from build123d import *

# Parameters (mm, degrees)
SKETCH1_W                = 20
SKETCH1_H                = 2
BOSS_EXTRUDE1_DEPTH      = 90
SKETCH2_W                = 2.795480737
SKETCH2_H                = 20
BOSS_EXTRUDE2_DEPTH      = 21
SKETCH3_W                = 3.5
SKETCH3_H                = 20
BOSS_EXTRUDE3_DEPTH      = 15
FILLET1_R                = 10.5
FILLET2_R                = 10
BOSS_EXTRUDE4_REACH      = 93.71
SKETCH4_W                = 1.5
SKETCH4_H                = 4
CUT_EXTRUDE1_REACH       = 57.51
SKETCH5_R                = 1.25
SKETCH5_R_2              = 3.5
CUT_EXTRUDE2_REACH       = 93.71
SKETCH6_R                = 0.925
SKETCH7_W                = 20
SKETCH7_H                = 8.6
CUT_EXTRUDE3_DEPTH       = 2.2
FILLET3_R                = 3.5
FILLET4_R                = 3.5
SKETCH8_W                = 3
SKETCH8_H                = 1
ZIPTIEHOLE_DEPTH         = 96.0181678
BOSS_EXTRUDE5_DEPTH      = 1.5
BOSS_EXTRUDE5_DEPTH_BACK = 1.5


# Some blends are built 0.0001 mm under size
with BuildPart() as part:
    # Sketch1 → Boss-Extrude1 (new body)
    with BuildSketch(Plane(origin=(0, 0, 0), x_dir=(0, 0, -1), z_dir=(1, 0, 0))):
        with Locations((10, 1)):
            Rectangle(SKETCH1_W, SKETCH1_H)
    extrude(amount=BOSS_EXTRUDE1_DEPTH)

    # Sketch2 → Boss-Extrude2 (add)
    with BuildSketch(Plane(origin=(0, 2, 0), x_dir=(1, 0, 0), z_dir=(0, 1, 0))):
        with Locations((44.997740369, 10)):
            Rectangle(SKETCH2_W, SKETCH2_H)
    extrude(amount=BOSS_EXTRUDE2_DEPTH)

    # Sketch3 → Boss-Extrude3 (add)
    with BuildSketch(Plane(origin=(0, 2, 0), x_dir=(1, 0, 0), z_dir=(0, 1, 0))):
        with Locations((88.25, 10)):
            Rectangle(SKETCH3_W, SKETCH3_H)
    extrude(amount=BOSS_EXTRUDE3_DEPTH)

    # Fillet1
    # the kernel refuses this fillet: 10.5 mm, written as the material it takes off along each edge
    with BuildSketch(Plane(origin=(72.645480737, 23, 0), x_dir=(0, 0, -1), z_dir=(-1, 0, 0)), Plane(origin=(17.35, 23, -20), x_dir=(0, 0, 1), z_dir=(1, 0, 0))) as fillet1_piece_1:
        with BuildLine():
            CenterArc((FILLET1_R, FILLET1_R), FILLET1_R, 180, 90)
            Line((0, FILLET1_R), (0, 0))
            Line((0, 0), (FILLET1_R, 0))
        make_face()
    extrude(amount=55.295480737, mode=Mode.SUBTRACT)

    # Fillet2
    fillet2_edges = [part.edges().sort_by_distance(p)[0] for p in [
        (88.25, 17, -20),
        (88.25, 17, 0),
    ]]
    fillet(fillet2_edges, radius=FILLET2_R - 0.0001)  # a hair under: the kernel refuses the full size

    # Boss-Extrude4: up to this face of the body (flat: up to its plane)
    boss_extrude4_end = Plane(part.part.faces().sort_by_distance((0, 1, -10))[0])
    # Sketch4 → Boss-Extrude4 (add, up to the picked face)
    with BuildSketch(Plane.ZY.offset(-86.5), mode=Mode.PRIVATE) as boss_extrude4_sk1:
        with Locations((-0.75, 4)):
            Rectangle(SKETCH4_W, SKETCH4_H)
    boss_extrude4_tool1 = split(extrude(boss_extrude4_sk1.sketch, amount=BOSS_EXTRUDE4_REACH, mode=Mode.PRIVATE), bisect_by=boss_extrude4_end, keep=Keep.BOTH, mode=Mode.PRIVATE)
    # Sketch4 → Boss-Extrude4 (add, up to the picked face)
    with BuildSketch(Plane.ZY.offset(-86.5), mode=Mode.PRIVATE) as boss_extrude4_sk2:
        with Locations((-19.25, 4)):
            Rectangle(SKETCH4_W, SKETCH4_H)
    boss_extrude4_tool2 = split(extrude(boss_extrude4_sk2.sketch, amount=BOSS_EXTRUDE4_REACH, mode=Mode.PRIVATE), bisect_by=boss_extrude4_end, keep=Keep.BOTH, mode=Mode.PRIVATE)
    add(boss_extrude4_tool1.solids().sort_by(Axis((86.5, 4, -0.75), (-1, 0, 0)))[0])
    add(boss_extrude4_tool2.solids().sort_by(Axis((86.5, 4, -19.25), (-1, 0, 0)))[0])

    # Sketch5 → Cut-Extrude1 (cut, up to next)
    with BuildSketch(Plane.ZY.offset(-43.6), mode=Mode.PRIVATE) as cut_extrude1_sk1:
        with Locations((-17.5, 12.2)):
            Circle(SKETCH5_R)
    cut_extrude1_tool1 = extrude(cut_extrude1_sk1.sketch, amount=-CUT_EXTRUDE1_REACH, mode=Mode.PRIVATE) & part.part
    # Sketch5 → Cut-Extrude1 (cut, up to next)
    with BuildSketch(Plane.ZY.offset(-43.6), mode=Mode.PRIVATE) as cut_extrude1_sk2:
        with Locations((-2.5, 12.2)):
            Circle(SKETCH5_R)
    cut_extrude1_tool2 = extrude(cut_extrude1_sk2.sketch, amount=-CUT_EXTRUDE1_REACH, mode=Mode.PRIVATE) & part.part
    # Sketch5 → Cut-Extrude1 (cut, up to next)
    with BuildSketch(Plane.ZY.offset(-43.6), mode=Mode.PRIVATE) as cut_extrude1_sk3:
        with Locations((-10, 12.2)):
            Circle(SKETCH5_R_2)
    cut_extrude1_tool3 = extrude(cut_extrude1_sk3.sketch, amount=-CUT_EXTRUDE1_REACH, mode=Mode.PRIVATE) & part.part
    add(cut_extrude1_tool1.solids().sort_by_distance((43.6, 12.2, -17.5))[0], mode=Mode.SUBTRACT)
    add(cut_extrude1_tool2.solids().sort_by_distance((43.6, 12.2, -2.5))[0], mode=Mode.SUBTRACT)
    add(cut_extrude1_tool3.solids().sort_by_distance((43.6, 12.2, -10))[0], mode=Mode.SUBTRACT)

    # Sketch6 → Cut-Extrude2 (cut, up to next)
    with BuildSketch(Plane.ZY.offset(-86.5), mode=Mode.PRIVATE) as cut_extrude2_sk1:
        with Locations((-10, 12.2)):
            Circle(SKETCH6_R)
    cut_extrude2_tool1 = extrude(cut_extrude2_sk1.sketch, amount=-CUT_EXTRUDE2_REACH, mode=Mode.PRIVATE) & part.part
    add(cut_extrude2_tool1.solids().sort_by_distance((86.5, 12.2, -10))[0], mode=Mode.SUBTRACT)

    # Sketch7 → Cut-Extrude3 (cut)
    with BuildSketch(Plane(origin=(90, 0, 0), x_dir=(0, 0, -1), z_dir=(1, 0, 0))):
        with Locations((10, 12.7)):
            Rectangle(SKETCH7_W, SKETCH7_H)
    extrude(amount=-CUT_EXTRUDE3_DEPTH, mode=Mode.SUBTRACT)

    # Fillet3
    fillet3_edges = [part.edges().sort_by_distance(p)[0] for p in [
        (21.8, 2, -1.5),
        (66.447740368, 2, -1.5),
        (66.447740368, 2, -18.5),
        (21.8, 2, -18.5),
    ]]
    fillet(fillet3_edges, radius=FILLET3_R)

    # Fillet4
    fillet4_edges = [part.edges().sort_by_distance(p)[0] for p in [
        (46.395480737, 2, -10),
        (46.395480737, 5.75, -1.5),
        (46.395480737, 3.025126266, -17.474873734),
        (46.395480737, 3.025126266, -2.525126266),
        (46.395480737, 5.75, -18.5),
    ]]
    fillet(fillet4_edges, radius=FILLET4_R)

    # Sketch8 → zipTieHole (cut, through all)
    with BuildSketch(Plane(origin=(0, 0, -20), x_dir=(-1, 0, 0), z_dir=(0, 0, -1))):
        with Locations((-26.4949995, 2)):
            Rectangle(SKETCH8_W, SKETCH8_H)
        with Locations((-70.5, 2.5)):
            Rectangle(SKETCH8_W, SKETCH8_H)
    extrude(amount=-ZIPTIEHOLE_DEPTH, mode=Mode.SUBTRACT)

    # Sketch10 → Boss-Extrude5 (add, two sides: drawn at the far end of the back side and taken through both)
    with BuildSketch(Plane(origin=(46.395480737, 5.5, -10), x_dir=(1, 0, 0), z_dir=(0, 0, 1)).offset(-BOSS_EXTRUDE5_DEPTH_BACK)):
        Polygon((7, -3.5), (0, 3.2), (0, -3.5), align=None)
    extrude(amount=BOSS_EXTRUDE5_DEPTH + BOSS_EXTRUDE5_DEPTH_BACK)


solid = part.part
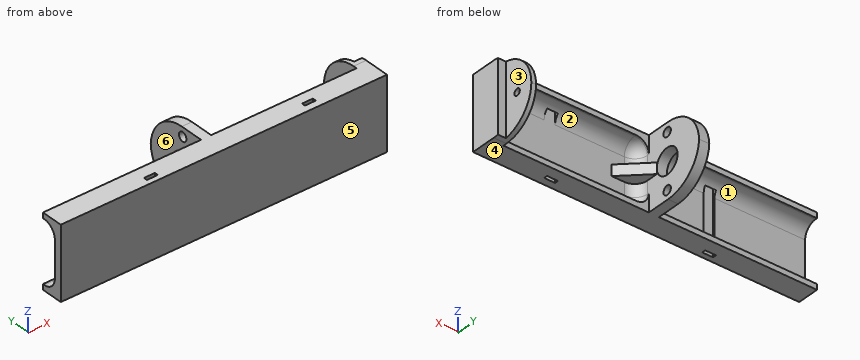
Model file for the job. Use its own axes, mm. Face numbers are marked on the shaded views. A direction names the side the tool comes from. Give positions to 0.01 mm unless a question says otherwise; leave off trailing zeros. Order: outer loops, then holes, each group sorted by start corner. A loop starts at its lowest first (then second) coordinate and runs counter-clockwise, first axis right, second up. Notation, with made-up numbers: M 28,48 L 55,48 A7 ccw 55,53 Z; hole C -27.75,86 d2. An arc over 180 degrees is marked long. Put each result on its own line as item: value. Start each with the question number.
(1) Pin check, flat tips, straight feed: pin 1 Ø12 at (y, z) = (13, -13.5) entering from -X; pin 2 Ø12 at (x, z) = (66, -14) entering from -Y; pin 3 Ø1.8 at (x, z) = (89, -9) entering from +Y; pin 4 Ø3 at (y, z) = (14.5, -8) entering from +X. Stop position of each tip, or through.
(2) Band-saw the part on A-A on x = 30.5. Give the cut face in (y, z).
(3) Pull direction Z, two halves, no side cores. Call the marked faces 4, 5 and 6: released by +Z, released by -Z, zero draft, split by the parting line, or undercut.
(4) Drill centre lines: L1, parallel to X at y = 14.5, z = -7.25; L2, parallel to X at y = 7.75, z = -11.75; L3, parallel to Y at x = 46.5, z = -3.75. Where is each one in solid material? Low to high. Write a range as [from, to].
(5) Band-saw the part on B-B on y = 20.5. Give the cut face in (x, z), then the cut area to 3 significant figures.
(6) Tool access for the marked faces 1, 2 and 3: list every direction of +Z, -Z, +X, -X, +Y, -Y with a clear straight run to the whole face (end or side of a thin tool).
Results below:
1. pin 1: stops at x = 43.6
1. pin 2: stops at y = 0
1. pin 3: stops at y = 8.4
1. pin 4: stops at x = 87.8
2. outline: M 0,-20 L 6,-20 L 6,-18.5 L 5.5,-18.5 A3.5 cw 2,-15 L 2,-5 A3.5 cw 5.5,-1.5 L 6,-1.5 L 6,0 L 0,0 Z
3. face 4: released by -Z
3. face 5: zero draft
3. face 6: undercut
4. L1: x = [43.6, 46.4], [86.5, 87.8]
4. L2: x = [43.6, 46.4], [86.5, 90]
4. L3: y = [0, 6]
5. outline: M 43.6,-16.3 L 46.4,-16.3 L 46.4,-3.7 L 43.6,-3.7 Z
5. area: 35.2 mm2
6. face 1: -X, +Y
6. face 2: +Y
6. face 3: +Z, -Z, +X, +Y
